For this review, take the finished solid that the model builds, in its own axes (mm). A direction names the side the tool comes from. Round coordinates to 2 decimals unless told otherwise and drop trailing zeros. Order: outer loops, then holes, each group sorted by start corner. A loop starts at its lowest first (then second) coordinate and runs counter-clockwise, first axis right, second up. Notation, with made-up numbers: M -18,86 L 2,86 A14 ccw 2,103 Z; hole C 46.25,-22 d3. An arc over 180 degrees is marked long. Use a Markdown table: item, result.
Autodesk Inventor part; units mm, degrees
ref_plane "YZ Plane" through (0, 0, 0) normal (1, 0, 0) x (0, 1, 0)
ref_plane "XZ Plane" through (0, 0, 0) normal (0, 1, 0) x (-1, 0, 0)
ref_plane "XY Plane" through (0, 0, 0) normal (0, 0, 1) x (1, 0, 0)
sketch "Sketch1" plane through (0, 0, 0) normal (0, 0, 1) x (1, 0, 0)
  circle A0 centre (0, 0) radius 2.5
  dimension "d0" = 5
extrude "Extrusion1" add sketch "Sketch1" along normal blind 250
sketch "Sketch2" plane through (0, 0, 250) normal (0, 0, 1) x (1, 0, 0)
  circle A0 centre (0, 0) radius 2.5
  line L0 (0, 0) -> (0, -25)
  line L1 (0, 0) -> (0, 25)
  line L2 (0, 25) -> (7.5, 25)
  line L3 (7.5, 25) -> (7.5, -25)
  line L4 (7.5, -25) -> (0, -25)
  point P0 (0, 0)
  dimension "d12" = 25
  dimension "d14" = 25
  dimension "d15" = 7.5
revolve "Revolution1" add sketch "Sketch2" angle 360 about axis through (0, 0, 250) along (0, 1, 0) picked at (1.6458, -0.1854) contours A0 L0 L1 | A0 L1 L2 L3 L4 L0
fillet "Fillet4" radius 7.5 1 edges at (-7.5, -25, 250)
properties part number "Threaded hammer"
Q1. Add section D-D (y = 20.5). Write out the cut boundary in (x, z), then the cut area to 3 significant figures.
Determined:
| item | result |
|---|---|
| outline | C 0,250 d15 |
| area | 177 mm^2 |
Q2. Wall thickness on line 1 along X through (y, z) = (0, 52.5); line 2 along Z through (x, y) = (-0.25, -9.5); line 3 along Z through (x, y) = (-6.25, -12.5): over which ranges is each line inside the solid? List them lowest first. Write a range as [from, to].
Determined:
| item | result |
|---|---|
| line 1 | x = [-2.5, 2.5] |
| line 2 | z = [242.5, 257.5] |
| line 3 | z = [245.85, 254.15] |
Q3. Clearance check with flat-ended pins moving along their axes: pin 1 (6 mm diameter, centred on x = 5, z = 179, fed in from -Y); pin 2 (1.5 mm diameter, centred on x = 4.5, y = 12.5, fed in from +Z); pin 3 (8 mm diameter, centred on y = 1, z = 162.5, fed in from +X). State where each tip first meets the part, or that it passes through.
Determined:
| item | result |
|---|---|
| pin 1 | stops at y = -1.5 |
| pin 2 | stops at z = 256.5 |
| pin 3 | stops at x = 2.5 |
Q4. Add section A-A (x = 0). Write out the cut boundary in (y, z).
Determined:
| item | result |
|---|---|
| outline | M -17.5,242.5 L -2.5,242.5 L -2.5,0 L 2.5,0 L 2.5,242.5 L 25,242.5 L 25,257.5 L -17.5,257.5 A7.5 ccw Z |
Q5. Add section B-B (y = 0). Write out the cut boundary in (x, z).
Determined:
| item | result |
|---|---|
| outline | M -2.5,0 L 2.5,0 L 2.5,242.93 A7.5 ccw long -2.5,242.93 Z |
Q6. Machinability: for faces 1 (the cylindrical face through (-0.54, 2.44, 119.76)), 2 (the flat face through (0, 25, 250)), which of the approach directions +Z, -Z, +X, -X, +Y, -Y give a long, thin tool a straight path to every point of the face, cutting with its end or side? Answer none if there is none.
Determined:
| item | result |
|---|---|
| face 1 | -Z |
| face 2 | +Z, -Z, +X, -X, +Y |
Q7. Add section C-C (z = 171). Write out the cut boundary in (x, y).
Determined:
| item | result |
|---|---|
| outline | C 0,0 d5 |
